from build123d import *

# Parameters (mm, degrees)
SKETCH1_W           = 100
SKETCH1_H           = 70
BOSS_EXTRUDE1_DEPTH = 10
SKETCH2_R           = 1.5
CUT_EXTRUDE1_DEPTH  = 5
SKETCH3_W           = 17.581829542
SKETCH3_H           = 1.056152304
SKETCH3_W_2         = 9.008357892
CUT_EXTRUDE2_DEPTH  = 5
FILLET1_R           = 1


with BuildPart() as part:
    # Sketch1 → Boss-Extrude1 (new body)
    with BuildSketch(Plane(origin=(0, 0, 0), x_dir=(1, 0, 0), z_dir=(0, 1, 0))):
        with Locations((50, 35)):
            Rectangle(SKETCH1_W, SKETCH1_H)
    extrude(amount=BOSS_EXTRUDE1_DEPTH)

    # Sketch2 → Cut-Extrude1 (cut)
    with BuildSketch(Plane.XZ):
        with Locations((14, -4)):
            Circle(SKETCH2_R)
        with Locations((14, -66)):
            Circle(SKETCH2_R)
        with Locations((91, -66)):
            Circle(SKETCH2_R)
        with Locations((91, -4)):
            Circle(SKETCH2_R)
    extrude(amount=-CUT_EXTRUDE1_DEPTH, mode=Mode.SUBTRACT)

    # Sketch3 → Cut-Extrude2 (cut)
    with BuildSketch(Plane.ZY):
        Polygon((-70, 6), (-70, 10), (0, 10), (0, 6), (-21, 6), (-21, 0), (-58.5, 0), (-58.5, 6), align=None)
        with Locations((-45.810029471, 3.819594483)):
            Rectangle(SKETCH3_W, SKETCH3_H, mode=Mode.SUBTRACT)
        with Locations((-29.035845809, 3.819594483)):
            Rectangle(SKETCH3_W_2, SKETCH3_H, mode=Mode.SUBTRACT)
    extrude(amount=-CUT_EXTRUDE2_DEPTH, mode=Mode.SUBTRACT)

    # Fillet1
    fillet1_edges = [part.edges().sort_by_distance(p)[0] for p in [
        (0, 3, -70),
        (0, 3, 0),
        (5, 8, -70),
        (5, 8, 0),
        (100, 5, -70),
        (100, 5, 0),
    ]]
    fillet(fillet1_edges, radius=FILLET1_R)


solid = part.part
The listing builds one solid part. Answer for the finished solid, in the listing's coordinates (mm). A direction names the side the tool comes from. Give positions to 0.01 mm unless a question says otherwise; leave off trailing zeros. Order: outer loops, then holes, each group sorted by start corner. A loop starts at its lowest first (then second) coordinate and runs counter-clockwise, first axis right, second up. Notation, with made-up numbers: (34, -7.75) -> (43, -7.75) arc R28 ccw to (43, 25.25) -> close; hole circle Ø11 at (80, -31). An arc over 180 degrees is marked (long way). Put each result on its own line as item: value.
Item 1: Given P1, Ø4, axis at x = 14, z = -4, coming from the -Y side; P2, Ø1.5, axis at x = 91.5, z = -66, coming from the -Y side; P3, Ø1.5, axis at x = 2.5, z = -46.5, coming from the +Y side; P4, Ø1.8, axis at x = 4, z = -10.5, coming from the +Y side, each flat-ended and moving along its own axis, determine where each tip first touches the part or whether it passes through.
Established:
P1: stops at y = 0
P2: stops at y = 5
P3: stops at y = 4.35
P4: stops at y = 6
Item 2: A cutting plane is placed at A-A on z = -49. Give the vertices of the cut face in (x, y), plus the area to 3 significant figures.
Established:
outline: (0, 3.29) -> (5, 3.29) -> (5, 0) -> (100, 0) -> (100, 10) -> (5, 10) -> (5, 4.35) -> (0, 4.35) -> close
area: 955 mm^2
Item 3: A cutting plane is placed at C-C on z = -66. Give the vertices of the cut face in (x, y).
Established:
outline: (0, 0) -> (12.5, 0) -> (12.5, 5) -> (15.5, 5) -> (15.5, 0) -> (89.5, 0) -> (89.5, 5) -> (92.5, 5) -> (92.5, 0) -> (100, 0) -> (100, 10) -> (5, 10) -> (5, 6) -> (0, 6) -> close
Item 4: For faces 1 (the face through (2, 3, -58.5)), 2 (the face through (2, 3.292, -29)), 3 (the face through (92.43, 2.46, -3.55)), determine the directions among +Z, -Z, +X, -X, +Y, -Y from which every point of the face is accessible in a straight line to the end or side of a thin tool.
Established:
face 1: -X, +Y, -Y
face 2: -X, -Y
face 3: -Y
Item 5: A cutting plane is placed at B-B on x = 91. Give the vertices of the cut face in (y, z), plus the area to 3 significant figures.
Established:
outline: (0, -70) -> (10, -70) -> (10, 0) -> (0, 0) -> (0, -2.5) -> (5, -2.5) -> (5, -5.5) -> (0, -5.5) -> (0, -64.5) -> (5, -64.5) -> (5, -67.5) -> (0, -67.5) -> close
area: 670 mm^2
Item 6: For a pull along Z with two mould halves and no side action, classify faces 4 (the face through (49, 5, 0)), 5 (the face through (52, 10, -35)), 6 (the face through (2, 4.348, -29)), 7 (the face through (2, 4.348, -46)) as released by +Z, released by -Z, zero draft, split by the parting line, or undercut.
Established:
face 4: released by +Z
face 5: zero draft
face 6: undercut
face 7: undercut
Item 7: Straight lines are drawn through the part: line 1 (Z direction, x = 91, y = 1.55); line 2 (X direction, y = 4.5, z = -54); line 3 (Z direction, x = 5.5, y = 9.25). For each, find the intervals that lie inside material, in ascending order.
Established:
line 1: z = -70 to -67.5, -64.5 to -5.5, -2.5 to 0
line 2: x = 5 to 100
line 3: z = -69.87 to -0.13
